Geometry check sheet. Reference: the model listing, model coordinates, mm. Give positions to 0.01 mm unless a question says otherwise; leave off trailing zeros. Write each loop counter-clockwise with the first axis right and the second up, starting at its lowest first coordinate (ties: lowest second). Pieces come first, ordered by that corner, then holes. Notation, with made-up numbers: M -8.5,27.5 L 26.5,27.5 A25 cw 26.5,45.5 Z; hole C 59.5,0 d2. An arc over 180 degrees is marked long. One line per item, written item: value. Start each with the question number.
1. Cross-section at C-C on x = 20. Record the cut outline in (y, z).
2. Scan lines: line 1 (Z direction, x = 10.25, y = 1.2); line 2 (Z direction, x = 19, y = 0.75); line 3 (X direction, y = 0.6, z = 59.5). Record each from-to range of solid material in increasing order.
3. Cross-section at A-A on z = 25. Record the cut outline in (x, y), then the cut area to 3 significant figures.
4. Gauge pin test, flat ends, axial feed: pin 1 (1 mm diameter, centred on y = 1, z = 24.5, fed in from -X); pin 2 (3.5 mm diameter, centred on x = 19, z = 9, fed in from +Y). Record the tip position at first contact, or that the pin passes through.
5. Cross-section at D-D on z = 49. Record the cut outline in (x, y).
6. Cross-section at B-B on y = 1.2. Count the separate pieces of the cut face and the enclosed holes in it, then the cut area to 3 significant figures.
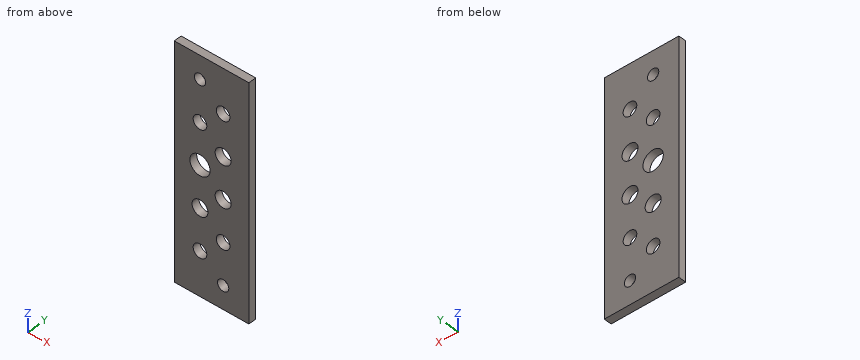
from build123d import *

# Parameters (mm, degrees)
F0_W     = 29
F0_H     = 90
F0_R     = 2.65
F0_R_2   = 3.1
F0_R_3   = 2.2
F0_R_4   = 3.95
F1_DEPTH = 3


with BuildPart() as f1:
    # F0 (on Front) → F1 (new body)
    with BuildSketch(Plane.XZ):
        with Locations((14.5, 45)):
            Rectangle(F0_W, F0_H)
        with Locations((10, 17)):
            Circle(F0_R, mode=Mode.SUBTRACT)
        with Locations((10, 33)):
            Circle(F0_R_2, mode=Mode.SUBTRACT)
        with Locations((19, 9)):
            Circle(F0_R_3, mode=Mode.SUBTRACT)
        with Locations((19, 25)):
            Circle(F0_R, mode=Mode.SUBTRACT)
        with Locations((19, 41)):
            Circle(F0_R_2, mode=Mode.SUBTRACT)
        with Locations((10, 49)):
            Circle(F0_R_4, mode=Mode.SUBTRACT)
        with Locations((10, 65)):
            Circle(F0_R, mode=Mode.SUBTRACT)
        with Locations((10, 81)):
            Circle(F0_R_3, mode=Mode.SUBTRACT)
        with Locations((19, 57)):
            Circle(F0_R_2, mode=Mode.SUBTRACT)
        with Locations((19, 73)):
            Circle(F0_R, mode=Mode.SUBTRACT)
    extrude(amount=-F1_DEPTH)


solid = f1.part
Report:
1. outline: M 0,0 L 3,0 L 3,7.04 L 0,7.04 Z; M 0,10.96 L 3,10.96 L 3,22.55 L 0,22.55 Z; M 0,27.45 L 3,27.45 L 3,38.07 L 0,38.07 Z; M 0,43.93 L 3,43.93 L 3,54.07 L 0,54.07 Z; M 0,59.93 L 3,59.93 L 3,70.55 L 0,70.55 Z; M 0,75.45 L 3,75.45 L 3,90 L 0,90 Z
2. line 1: z = 0 to 14.36, 19.64 to 29.91, 36.09 to 45.06, 52.94 to 62.36, 67.64 to 78.81, 83.19 to 90
2. line 2: z = 0 to 6.8, 11.2 to 22.35, 27.65 to 37.9, 44.1 to 53.9, 60.1 to 70.35, 75.65 to 90
2. line 3: x = 0 to 17.17, 20.83 to 29
3. outline: M 0,0 L 16.35,0 L 16.35,3 L 0,3 Z; M 21.65,0 L 29,0 L 29,3 L 21.65,3 Z
3. area: 71.1 mm^2
4. pin 1: stops at x = 0
4. pin 2: passes through
5. outline: M 0,0 L 6.05,0 L 6.05,3 L 0,3 Z; M 13.95,0 L 29,0 L 29,3 L 13.95,3 Z
6. separate pieces: 1
6. enclosed holes: 10
6. area: 2,350 mm^2
